Check sheet for the modelled part. Datum: model origin and axes. Units: mm. A direction names the side the tool comes from. Round coordinates to 2 decimals unless told otherwise and drop trailing zeros. Write each loop counter-clockwise with the first axis right and the second up, starting at its lowest first coordinate (ties: lowest second). Pieces come first, ordered by that corner, then holes. Notation, with made-up numbers: M 69,1 L 124,1 A34 ccw 124,32 Z; hole C 25,72 d2. An arc over 180 degrees is marked long. Put each result on its own line as item: value.
```python
from build123d import *

# Parameters (mm, degrees)
AXLE_SUPPORT_PLATE_R   = 7.030128061
AXLE_SUPPORT_PLATE_R_2 = 2.159
AXLE_SUPPORT_PLATE_W   = 6.35
AXLE_SUPPORT_PLATE_H   = 6.35
BOSS_EXTRUDE1_DEPTH    = 6.35


with BuildPart() as part:
    # Axle Support Plate → Boss-Extrude1 (new body)
    with BuildSketch(Plane(origin=(0, 0, 0), x_dir=(1, 0, 0), z_dir=(0, 1, 0))):
        Polygon((31.160128061, -180.975), (31.160128061, -13.380128061), (113.120256121, -13.380128061), (113.120256121, -3.175), (125.820256121, -3.175), (125.820256121, 3.175), (113.120256121, 3.175), (113.120256121, 13.380128061), (31.160128061, 13.380128061), (31.160128061, 158.160128061), (0, 158.160128061), (0, -187.325), (6.35, -187.325), (6.35, -180.975), (12.7, -180.975), (12.7, -175.440000021), (10.659000018, -175.440000021), (10.659000018, -172.539999979), (12.7, -172.539999979), (12.7, -167.005), (17.018, -167.005), (17.018, -172.539999979), (19.058999982, -172.539999979), (19.058999982, -175.440000021), (17.018, -175.440000021), (17.018, -180.975), (23.368, -180.975), (23.368, -187.325), (29.718, -187.325), (29.718, -180.975), align=None)
        with Locations(Location((19.05, 146.05, 0), (0, 0, 270))):
            Circle(AXLE_SUPPORT_PLATE_R, mode=Mode.SUBTRACT)
        with Locations(Location((19.05, -146.05, 0), (0, 0, 90))):
            Circle(AXLE_SUPPORT_PLATE_R, mode=Mode.SUBTRACT)
        with Locations(Location((9.525, 65.659, 0), (0, 0, 270))):
            Circle(AXLE_SUPPORT_PLATE_R_2, mode=Mode.SUBTRACT)
        with Locations(Location((9.525, -65.659, 0), (0, 0, 90))):
            Circle(AXLE_SUPPORT_PLATE_R_2, mode=Mode.SUBTRACT)
        with Locations((9.525, -77.343)):
            Rectangle(AXLE_SUPPORT_PLATE_W, AXLE_SUPPORT_PLATE_H, mode=Mode.SUBTRACT)
        with Locations((9.525, 77.343)):
            Rectangle(AXLE_SUPPORT_PLATE_W, AXLE_SUPPORT_PLATE_H, mode=Mode.SUBTRACT)
        with BuildLine():
            Line((38.190256121, 7.030128061), (76.290256121, 7.030128061))
            ThreePointArc((76.290256121, 7.030128061), (83.320384182, 0), (76.290256121, -7.030128061))
            Line((76.290256121, -7.030128061), (38.190256121, -7.030128061))
            ThreePointArc((38.190256121, -7.030128061), (31.160128061, 0), (38.190256121, 7.030128061))
        make_face(mode=Mode.SUBTRACT)
    extrude(amount=BOSS_EXTRUDE1_DEPTH)


solid = part.part
```
1. Cross-section at B-B (x = 58). Enter the section's corners in (y, z), then the cut area to 3 significant figures.
Computed values:
outline: M 0,-13.38 L 6.35,-13.38 L 6.35,-7.03 L 0,-7.03 Z; M 0,7.03 L 6.35,7.03 L 6.35,13.38 L 0,13.38 Z
area: 80.6 mm2
2. Depth check by flat-ended pin: pin 1 Ø0.9 at (y, z) = (3, 174.5) entering from +X; pin 2 Ø1.9 at (y, z) = (2.5, -6) entering from +X; pin 3 Ø3 at (x, y) = (8.5, 2.5) entering from +Z (3 decimals). Enter the tip coordinate at first touch or a pass-through.
Computed values:
pin 1: stops at x = 31.16
pin 2: stops at x = 113.12
pin 3: stops at z = 180.975
3. Cross-section at D-D (y = 2.25). Count the separate pieces of the cut face and the enclosed holes in it, then the cut area to 3 significant figures.
Computed values:
separate pieces: 1
enclosed holes: 7
area: 11,700 mm2
4. Cross-section at A-A (z = -146.05). Enter the section's corners in (x, y), then the cut area to 3 significant figures.
Computed values:
outline: M 0,0 L 12.02,0 L 12.02,6.35 L 0,6.35 Z; M 26.08,0 L 31.16,0 L 31.16,6.35 L 26.08,6.35 Z
area: 109 mm2
5. Access from +Z, -Z, +X, -X, +Y, -Y to the whole of each face (thin tool, end or side, straight path). Record for faces 4 (the flat face through (58, 3, 7.03)), 5 (the flat face through (73, 3, -13.38)), 6 (the flat face through (113.12, 3, 8)), 7 (the flat face through (23.368, 3, 184)).
Computed values:
face 4: +Y, -Y
face 5: -Z, +X, +Y, -Y
face 6: +Z, +X, +Y, -Y
face 7: +Z, +Y, -Y
6. Release check for a two-part mould opening along Z. For faces 1 (the flat face through (31.16, 3, -85)), 2 (the flat face through (72, 3, 13.38)), 3 (the flat face through (9, 3, -80.518)) record: +Z half, -Z half, draft (parallel to the pull), parting line (faces both ways), or undercut.
Computed values:
face 1: draft
face 2: +Z half
face 3: undercut
7. Cross-section at C-C (x = 92.5). Enter the section's corners in (y, z).
Computed values:
outline: M 0,-13.38 L 6.35,-13.38 L 6.35,13.38 L 0,13.38 Z
8. Scan lines: probe 1 along Z at (x, y) = (9.5, 2) (3 decimals); probe 2 along Z at (x, y) = (53, 6.25); probe 3 along Z at (x, y) = (20.5, 0.5) (3 decimals). Record each from-to range of solid material in increasing order.
Computed values:
probe 1: z = -158.16 to -80.518, -74.168 to -67.818, -63.5 to 63.5, 67.818 to 74.168, 80.518 to 180.975
probe 2: z = -13.38 to -7.03, 7.03 to 13.38
probe 3: z = -158.16 to -152.929, -139.171 to 139.171, 152.929 to 180.975
